from build123d import *

# Parameters (mm, degrees)
SKETCH_1_R           = 11
EXTRUDE_1_DEPTH      = 11
SKETCH_2_R           = 8.2
CUT_EXTRUDE_1_DEPTH  = 9.35
SKETCH_4_R           = 3.4
EXTRUDE_2_DEPTH      = 17.75
SKETCH_5_R           = 1.5
CUT_EXTRUDE_4_DEPTH  = 25.75
SKETCH_6_R           = 13.6
SKETCH_6_R_2         = 11
EXTRUDE_4_DEPTH      = 2.95
EXTRUDE_4_DEPTH_BACK = 13.95


with BuildPart() as part:
    # ｽｹｯﾁ1 → ﾎﾞｽ - 押し出し1 (new body)
    with BuildSketch(Plane(origin=(0, 0, 0), x_dir=(0, 0, -1), z_dir=(1, 0, 0))):
        Circle(SKETCH_1_R)
    extrude(amount=EXTRUDE_1_DEPTH)

    # ｽｹｯﾁ2 → ｶｯﾄ - 押し出し1 (cut)
    with BuildSketch(Plane(origin=(11, 0, 0), x_dir=(0, 0, -1), z_dir=(1, 0, 0))):
        Circle(SKETCH_2_R)
    extrude(amount=-CUT_EXTRUDE_1_DEPTH, mode=Mode.SUBTRACT)

    # ｽｹｯﾁ4 → ﾎﾞｽ - 押し出し2 (add)
    with BuildSketch(Plane(origin=(1.65, 0, 0), x_dir=(0, 0, -1), z_dir=(1, 0, 0))):
        Circle(SKETCH_4_R)
    extrude(amount=EXTRUDE_2_DEPTH)

    # ｽｹｯﾁ5 → ｶｯﾄ - 押し出し4 (cut)
    with BuildSketch(Plane(origin=(19.4, 0, 0), x_dir=(0, 0, -1), z_dir=(1, 0, 0))):
        Circle(SKETCH_5_R)
    extrude(amount=-CUT_EXTRUDE_4_DEPTH, mode=Mode.SUBTRACT)

    # ｽｹｯﾁ6 → ﾎﾞｽ - 押し出し4 (add, two sides)
    with BuildSketch(Plane.ZY) as extrude_4_sk:
        Circle(SKETCH_6_R)
        Circle(SKETCH_6_R_2, mode=Mode.SUBTRACT)
    extrude(amount=EXTRUDE_4_DEPTH)
    extrude(extrude_4_sk.sketch, amount=-EXTRUDE_4_DEPTH_BACK)


solid = part.part
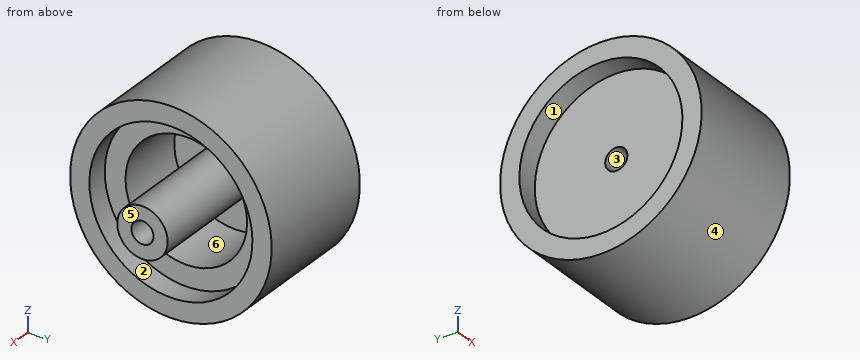
The model under review builds one solid part; all positions refer to its coordinate system, in mm. Face numbers are marked on the shaded views. A direction names the side the tool comes from. Give positions to 0.01 mm unless a question says otherwise; leave off trailing zeros. Loops run counter-clockwise (first coordinate to the right, second up) from the corner with the lowest first, then second, coordinate; pieces in that order, holes last. Notation, with made-up numbers: (-29.5, 21.25) -> (-15.5, 21.25) arc R8 cw to (-15.5, 29.25) -> close; hole circle Ø2 at (46.25, 24). An arc over 180 degrees is marked (long way). Write each question's results on one line, items separated by ' | '.
1) Take a section at C-C, the plane x = 17. Give the boundary of the cut face in (y, z).
Conclusion:
outline: circle Ø6.8 at (0, 0); hole circle Ø3 at (0, 0)
2) Draft analysis for pull direction Y (two halves, no side actions). For the marked faces 4, 5 and 6, state which applies: pulls with the +Y half, pulls with the -Y half, needs draft (parallel to the pull), parting line crosses it, or undercut.
Conclusion:
face 4: parting line crosses it | face 5: needs draft | face 6: undercut
3) For line 1 along Y through (x, z) = (6.25, 0); line 2 along Y through (x, z) = (12.9, 0); line 3 along Z through (x, y) = (10, 2.5), list the stretches that pass through material, from the lowest coordinate up. Write a range as from..to.
Conclusion:
line 1: y = -13.6..-8.2, -3.4..-1.5, 1.5..3.4, 8.2..13.6 | line 2: y = -13.6..-11, -3.4..-1.5, 1.5..3.4, 11..13.6 | line 3: z = -13.37..-7.81, -2.3..2.3, 7.81..13.37
4) Tool access review of the marked faces 1, 2 and 3: name each direction out of +Z, -Z, +X, -X, +Y, -Y from which nothing blocks a thin tool from reaching the whole face with its end or side.
Conclusion:
face 1: -X | face 2: +X | face 3: +X, -X
5) Take a section at A-A, the plane z = 0. Give the boundary of the cut face in (x, y).
Conclusion:
outline: (-2.95, -13.6) -> (13.95, -13.6) -> (13.95, -11) -> (11, -11) -> (11, -8.2) -> (1.65, -8.2) -> (1.65, -3.4) -> (19.4, -3.4) -> (19.4, -1.5) -> (0, -1.5) -> (0, -11) -> (-2.95, -11) -> close; (-2.95, 11) -> (0, 11) -> (0, 1.5) -> (19.4, 1.5) -> (19.4, 3.4) -> (1.65, 3.4) -> (1.65, 8.2) -> (11, 8.2) -> (11, 11) -> (13.95, 11) -> (13.95, 13.6) -> (-2.95, 13.6) -> close
6) Insertion check: pin 1 Ø1 at (x, y) = (9, 0.5) entering from -Z; pin 2 Ø10 at (x, y) = (11.5, 7) entering from -Z; pin 3 Ø1.5 at (x, z) = (6.5, 8) entering from +Y; pin 4 Ø10 at (y, z) = (5.5, -11) entering from +X. Each pin has a flat end and moves straight along its axis. Give the tip position at first contact, or say it passes through.
Conclusion:
pin 1: stops at z = -13.6 | pin 2: stops at z = -13.45 | pin 3: stops at y = 11.51 | pin 4: stops at x = 13.95
7) Take a section at D-D, the plane z = 8.75. Give the boundary of the cut face in (x, y), plus the area to 3 significant figures.
Conclusion:
outline: (-2.95, -10.41) -> (13.95, -10.41) -> (13.95, -6.67) -> (11, -6.67) -> (11, 6.67) -> (13.95, 6.67) -> (13.95, 10.41) -> (-2.95, 10.41) -> (-2.95, 6.67) -> (0, 6.67) -> (0, -6.67) -> (-2.95, -6.67) -> close | area: 273 mm^2
